from build123d import *

# Parameters (mm, degrees)
SKETCH_1_W      = 43
SKETCH_1_H      = 20
EXTRUDE_1_DEPTH = 1.6
SKETCH_2_R      = 8.272930051
EXTRUDE_2_DEPTH = 13.4
FILLET_1_R      = 1.6
SKETCH_9_W      = 10.16
SKETCH_9_H      = 2.54
EXTRUDE_3_DEPTH = 1.6


with BuildPart() as part:
    # 스케치1 → 보스-돌출1 (new body)
    with BuildSketch(Plane(origin=(0, 0, 0), x_dir=(1, 0, 0), z_dir=(0, 1, 0))):
        Rectangle(SKETCH_1_W, SKETCH_1_H)
    extrude(amount=EXTRUDE_1_DEPTH)

    # 스케치2 → 보스-돌출2 (add)
    with BuildSketch(Plane(origin=(0, 1.6, 0), x_dir=(1, 0, 0), z_dir=(0, 1, 0))):
        with Locations(Location((-10.75, 0, 0), (0, 0, 90))):
            Circle(SKETCH_2_R)
        with Locations(Location((10.75, 0, 0), (0, 0, 90))):
            Circle(SKETCH_2_R)
    extrude(amount=EXTRUDE_2_DEPTH)

    # 필렛1
    fillet_1_edges = [part.edges().sort_by_distance(p)[0] for p in [
        (-10.75, 15, 8.272930051),
        (10.75, 15, 8.272930051),
    ]]
    fillet(fillet_1_edges, radius=FILLET_1_R)

    # 스케치9 → 보스-돌출3 (add)
    with BuildSketch(Plane.XZ):
        with Locations((-1.27, -8.59488099)):
            Rectangle(SKETCH_9_W, SKETCH_9_H)
    extrude(amount=EXTRUDE_3_DEPTH)


solid = part.part
Read the model definition and answer for the solid it produces. Units are mm, in the model's axes. A direction names the side the tool comes from. Round coordinates to 2 decimals unless told otherwise and drop trailing zeros. Write each loop counter-clockwise with the first axis right and the second up, starting at its lowest first coordinate (ties: lowest second). Pieces come first, ordered by that corner, then holes.
1. Straight lines are drawn through the part: L1, parallel to Y at x = 18.5, z = -3.75; L2, parallel to X at y = 12.5, z = 1; L3, parallel to Z at x = 10.5, y = 3.75. For each, find the intervals that lie inside material, in ascending order.
2. The part is cut by section C-C, the plane z = 0. Determine the outline of the cut face in (x, y).
3. Determine the mould class of faces 6 (the face through (3.81, -1, -9)), 7 (the face through (0, 1.6, 0)), 8 (the face through (-1, -1.6, -9)) for opening direction X: pulls with the +X half, pulls with the -X half, needs draft (parallel to the pull), parting line crosses it, or undercut.
4. Which of the six approach directions +Z, -Z, +X, -X, +Y, -Y give full straight-line access (tool end or side, diameter ignored) to faces 1 (the face through (-1, -1, -7.325)), 2 (the face through (-1, -1, -9.865)), 3 (the face through (21.5, 1, 0)), 4 (the face through (3.774, 7.417, -4.447)), 5 (the face through (-6.35, -1, -9))?
5. Given pin 1 Ø0.5 at (y, z) = (-1, -8.5) entering from +X; pin 2 Ø10 at (x, z) = (9.5, 1.5) entering from -Y; pin 3 Ø1 at (x, y) = (-8.5, 2.5) entering from +Z, each flat-ended and moving along its own axis, determine where each tip first touches the part or whether it passes through.
6. The part is cut by section A-A, the plane x = -10.75. Determine the outline of the cut face in (y, z), then the cut area to 3 significant figures.
7. The part is cut by section B-B, the plane y = 2.75. Determine the outline of the cut face in (x, z).
8. The part is cut by section D-D, the plane x = 0. Determine the outline of the cut face in (y, z).
Values:
1. L1: y = 0 to 1.6
1. L2: x = -18.96 to -2.54, 2.54 to 18.96
1. L3: z = -8.27 to 8.27
2. outline: (-21.5, 0) - (21.5, 0) - (21.5, 1.6) - (19.02, 1.6) - (19.02, 13.4) arc R1.6 ccw to (17.42, 15) - (4.08, 15) arc R1.6 ccw to (2.48, 13.4) - (2.48, 1.6) - (-2.48, 1.6) - (-2.48, 13.4) arc R1.6 ccw to (-4.08, 15) - (-17.42, 15) arc R1.6 ccw to (-19.02, 13.4) - (-19.02, 1.6) - (-21.5, 1.6) - close
3. face 6: pulls with the +X half
3. face 7: undercut
3. face 8: needs draft
4. face 1: +Z, +X, -X, -Y
4. face 2: -Z, +X, -X, -Y
4. face 3: +Z, -Z, +X, +Y, -Y
4. face 4: +Y
4. face 5: +Z, -Z, -X, -Y
5. pin 1: stops at x = 3.81
5. pin 2: stops at y = 0
5. pin 3: stops at z = 8.09
6. outline: (0, -10) - (1.6, -10) - (1.6, -8.27) - (13.4, -8.27) arc R1.6 ccw to (15, -6.67) - (15, 6.67) arc R1.6 ccw to (13.4, 8.27) - (1.6, 8.27) - (1.6, 10) - (0, 10) - close
6. area: 253 mm2
7. outline: circle Ø16.55 at (-10.75, 0); circle Ø16.55 at (10.75, 0)
8. outline: (-1.6, -9.86) - (0, -9.86) - (0, -10) - (1.6, -10) - (1.6, 10) - (0, 10) - (0, -7.32) - (-1.6, -7.32) - close
